Geometry: final body of the model. Coordinates: model frame, mm. A direction names the side the tool comes from. Round coordinates to 2 decimals unless told otherwise and drop trailing zeros. Order: outer loops, then holes, each group sorted by start corner. A loop starts at its lowest first (then second) coordinate and runs counter-clockwise, first axis right, second up. Notation, with made-up numbers: (-23.75, 38.25) -> (-2.75, 38.25) arc R35 ccw to (-2.75, 76.25) -> close; hole circle Ø2 at (14.5, 17.25). An arc over 180 degrees is marked (long way). Put each result on its own line as item: value.
```python
from build123d import *

# Parameters (mm, degrees)
F0_W     = 25.4
F0_H     = 10.9855
F1_DEPTH = 6.35


with BuildPart() as f1:
    # F0 (on Top) → F1 (new body)
    with BuildSketch(Plane.XY):
        with Locations((0.85008, -1.236201)):
            Rectangle(F0_W, F0_H)
        with BuildLine():
            Line((-4.7625, 1.524), (-4.7625, 0))
            Line((-4.7625, 0), (-4.7625, -1.524))
            ThreePointArc((-4.7625, -1.524), (-6.35, -3.1115), (-7.9375, -1.524))
            Line((-7.9375, -1.524), (-7.9375, 0))
            Line((-7.9375, 0), (-7.9375, 1.524))
            ThreePointArc((-7.9375, 1.524), (-6.35, 3.1115), (-4.7625, 1.524))
        make_face(mode=Mode.SUBTRACT)
        with BuildLine():
            Line((7.9375, 1.524), (7.9375, 0))
            Line((7.9375, 0), (7.9375, -1.524))
            ThreePointArc((7.9375, -1.524), (6.35, -3.1115), (4.7625, -1.524))
            Line((4.7625, -1.524), (4.7625, 0))
            Line((4.7625, 0), (4.7625, 1.524))
            ThreePointArc((4.7625, 1.524), (6.35, 3.1115), (7.9375, 1.524))
        make_face(mode=Mode.SUBTRACT)
    extrude(amount=F1_DEPTH)


solid = f1.part
```
1. Cut plane D-D on x = -6.5. Return loops of the section in (y, z), and give its area (3 significant figures).
Ans:
outline: (-6.73, 0) -> (-3.1, 0) -> (-3.1, 6.35) -> (-6.73, 6.35) -> close; (3.1, 0) -> (4.26, 0) -> (4.26, 6.35) -> (3.1, 6.35) -> close
area: 30.3 mm²
2. Set-up query: faces 5 (the face through (13.55, -1, 3)), 6 (the face through (6.32, 3.11, 3.13)). Return all of +Z, -Z, +X, -X, +Y, -Y with unobstructed straight access to the full face (end or side cutting, diameter ignored); none if empty.
Ans:
face 5: +Z, -Z, +X, +Y, -Y
face 6: +Z, -Z
3. Cut plane B-B on z = 0.75. State how many separate pieces and enclosed holes the cut face has, and give its area (3 significant figures).
Ans:
separate pieces: 1
enclosed holes: 2
area: 244 mm²
4. Cut plane A-A on y = -0.5. Return loops of the section in (x, z).
Ans:
outline: (-11.85, 0) -> (-7.94, 0) -> (-7.94, 6.35) -> (-11.85, 6.35) -> close; (-4.76, 0) -> (4.76, 0) -> (4.76, 6.35) -> (-4.76, 6.35) -> close; (7.94, 0) -> (13.55, 0) -> (13.55, 6.35) -> (7.94, 6.35) -> close
5. Draft query along Y for faces 1 (the face through (1, -1, 0)), 2 (the face through (7.938, 0, 3)), 3 (the face through (1, 4.257, 3)), 4 (the face through (6.38, -3.11, 3.13)). Return one class per face: +Y half, -Y half, draft (parallel to the pull), parting line (faces both ways), or undercut.
Ans:
face 1: draft
face 2: undercut
face 3: +Y half
face 4: undercut
6. Cut plane C-C on x = 6.35. Return loops of the section in (y, z).
Ans:
outline: (-6.73, 0) -> (-3.11, 0) -> (-3.11, 6.35) -> (-6.73, 6.35) -> close; (3.11, 0) -> (4.26, 0) -> (4.26, 6.35) -> (3.11, 6.35) -> close
7. Material intervals for probe 1 along X at (y, z) = (-1.5, 0.5); probe 2 along X at (y, z) = (2.25, 3.75); probe 3 along Y at (x, z) = (-6, 6.25), sorted ascending.
Ans:
probe 1: -11.85 to -7.94, -4.76 to 4.76, 7.94 to 13.55
probe 2: -11.85 to -7.76, -4.94 to 4.94, 7.76 to 13.55
probe 3: -6.73 to -3.07, 3.07 to 4.26
